```python
from build123d import *

# Parameters (mm, degrees)
F0_W     = 35
F0_H     = 31
F0_W_2   = 13.5
F0_H_2   = 8
F0_W_3   = 29.5
F0_H_3   = 35
F1_DEPTH = 5


with BuildPart() as f1:
    # F0 (on Front) → F1 (new body)
    with BuildSketch(Plane.XZ):
        with Locations((-52.75, 0)):
            Rectangle(F0_W, F0_H)
        Polygon((-14.75, 30.5), (-35.25, 30.5), (-35.25, 15.5), (-35.25, -15.5), (-35.25, -30.5), (-14.75, -30.5), (14.75, -30.5), (35.25, -30.5), (35.25, -15.5), (35.25, 15.5), (35.25, 30.5), (14.75, 30.5), align=None)
        with Locations((-21.5, -19.5)):
            Rectangle(F0_W_2, F0_H_2, mode=Mode.SUBTRACT)
        with Locations((21.5, -19.5)):
            Rectangle(F0_W_2, F0_H_2, mode=Mode.SUBTRACT)
        with Locations((-21.5, 19.5)):
            Rectangle(F0_W_2, F0_H_2, mode=Mode.SUBTRACT)
        with Locations((21.5, 19.5)):
            Rectangle(F0_W_2, F0_H_2, mode=Mode.SUBTRACT)
        with Locations((0, 48)):
            Rectangle(F0_W_3, F0_H_3)
        with Locations((0, -48)):
            Rectangle(F0_W_3, F0_H_3)
        with Locations((52.75, 0)):
            Rectangle(F0_W, F0_H)
    extrude(amount=F1_DEPTH)


solid = f1.part
```
The listing builds one solid part. Answer for the finished solid, in the listing's coordinates (mm). A direction names the side the tool comes from. Round coordinates to 2 decimals unless told otherwise and drop trailing zeros. Loops run counter-clockwise (first coordinate to the right, second up) from the corner with the lowest first, then second, coordinate; pieces in that order, holes last. Notation, with made-up numbers: (-9, -5) - (24, -5) arc R23 ccw to (24, 17) - close; hole circle Ø5 at (47, 23). An arc over 180 degrees is marked (long way). Use one line per item in the form item = value. Start each with the question number.
1. The part is cut by section A-A on z = -18.5. Determine the outline of the cut face in (x, y), then the cut area to 4 significant figures.
2. The part is cut by section C-C on x = 32.5. Determine the outline of the cut face in (y, z), then the cut area to 3 significant figures.
3. The part is cut by section D-D on z = 37. Determine the outline of the cut face in (x, y).
4. A tool of negligible diameter and unlimited length cuts with its end or side. For faces 1 (the face through (53, -2, 15.5)), 2 (the face through (25, -2, -30.5)), 3 (the face through (-14.75, -2, -20)), 4 (the face through (-35.25, -2, -23)), from which of +Z, -Z, +X, -X, +Y, -Y can it reach the whole face along a straight path? Write none if from no direction.
5. For a pull along X with two mould halves and no side action, classify faces 5 (the face through (14.75, -2, -20)), 6 (the face through (53, -2, -15.5)), 7 (the face through (21, -2, -15.5)), 8 (the face through (35.25, -2, 23)) as pulls with the +X half, pulls with the -X half, needs draft (parallel to the pull), parting line crosses it, or undercut.
6. Consider line 1 (Z direction, x = 17.5, y = -1.25); line 2 (X direction, y = -3.3, z = 44.5); line 3 (Z direction, x = 53, y = -2). Determine where each line is inside the solid, lowest interval first. Write a range as [from, to].
7. Given pin 1 Ø2.5 at (y, z) = (-2, 18) entering from +X; pin 2 Ø2.5 at (x, y) = (-59.5, -3.5) entering from -Z; pin 3 Ø1.5 at (y, z) = (-3.5, -50) entering from -X; pin 4 Ø5 at (x, z) = (34, 8.5) entering from +Y, each flat-ended and moving along its own axis, determine where each tip first touches the part or whether it passes through.
8. The part is cut by section B-B on y = -3.45. Give the number of separate pieces and of enclosed holes in the cut face, then the cut area to 3 significant figures.
Geometry check:
q1.outline = (-35.25, -5) - (-28.25, -5) - (-28.25, 0) - (-35.25, 0) - close; (-14.75, -5) - (14.75, -5) - (14.75, 0) - (-14.75, 0) - close; (28.25, -5) - (35.25, -5) - (35.25, 0) - (28.25, 0) - close
q1.area = 217.5 mm^2
q2.outline = (-5, -30.5) - (0, -30.5) - (0, 30.5) - (-5, 30.5) - close
q2.area = 305 mm^2
q3.outline = (-14.75, -5) - (14.75, -5) - (14.75, 0) - (-14.75, 0) - close
q4.face_1 = +Z, +X, +Y, -Y
q4.face_2 = -Z, +X, +Y, -Y
q4.face_3 = +Y, -Y
q4.face_4 = -Z, -X, +Y, -Y
q5.face_5 = undercut
q5.face_6 = needs draft
q5.face_7 = undercut
q5.face_8 = pulls with the +X half
q6.line_1 = [-30.5, -23.5], [-15.5, 15.5], [23.5, 30.5]
q6.line_2 = [-14.75, 14.75]
q6.line_3 = [-15.5, 15.5]
q7.pin_1 = 35.25
q7.pin_2 = -15.5
q7.pin_3 = -14.75
q7.pin_4 = 0
q8.separate_pieces = 1
q8.enclosed_holes = 4
q8.area = 8,100 mm^2
